```python
from build123d import *

# Parameters (mm, degrees)
EXTRUDE1_DEPTH  = 1.5875
LPATTERN2_COUNT = 5
LPATTERN2_PITCH = 0.79375


with BuildPart() as part:
    # Sketch1 → Extrude1 (new body, symmetric)
    with BuildSketch(Plane(origin=(0, 0, 0), x_dir=(1, 0, 0), z_dir=(0, 1, 0))):
        Polygon((0, 5.040989538), (-4.365625, 2.520494769), (-4.365625, -2.520494769), (0, -5.040989538), (4.365625, -2.520494769), (4.365625, 2.520494769), align=None)
    extrude(amount=EXTRUDE1_DEPTH, both=True)

    # Sketch2 → Cut-Revolve1 (revolve, cut)
    with BuildSketch(Plane(origin=(0, 0, 0), x_dir=(0, 0, -1), z_dir=(1, 0, 0))):
        Polygon((4.365625, 1.5875), (5.040989538, 1.5875), (5.040989538, 1.272572344), align=None)
    revolve(axis=Axis((0, 1.421434714, 0), (0, -1, 0)), mode=Mode.SUBTRACT)

    # Sketch3 → Cut-Revolve3 (revolve, cut)
    with BuildSketch(Plane.XY):
        Polygon((1.65317021, 1.48828125), (1.65317021, 1.5875), (0, 1.5875), (0, 0.79375), (1.65317021, 0.79375), (2.0828, 1.041796875), (2.0828, 1.240234375), align=None)
    cut_revolve3 = revolve(axis=Axis((0, 1.642101285, 0), (0, -1, 0)), mode=Mode.SUBTRACT)

    # LPattern2: Cut-Revolve3 ×5
    with Locations(*[(0, -i * LPATTERN2_PITCH, 0) for i in range(1, LPATTERN2_COUNT)]):
        add(cut_revolve3, mode=Mode.SUBTRACT)

    # Sketch4 → Cut-Revolve4 (revolve, cut)
    with BuildSketch(Plane.XY):
        Polygon((1.867985105, 1.364257812), (1.996874042, 1.5875), (1.65317021, 1.5875), (1.65317021, 1.48828125), align=None)
    revolve(axis=Axis((0, 1.785862642, 0), (0, -1, 0)), mode=Mode.SUBTRACT)

    # Sketch12 → Revolve1 (revolve)
    with BuildSketch(Plane(origin=(0, 0, 0), x_dir=(0, 0, -1), z_dir=(1, 0, 0))):
        Polygon((2.70049032, -1.7145), (3.749364928, -1.7145), (4.7625, -1.985968724), (4.631019925, -2.476659044), (3.617884853, -2.20519032), (2.0828, -2.20519032), (2.0828, -1.5875), (2.70049032, -1.5875), align=None)
    revolve(axis=Axis((0, 1.620050577, 0), (0, -1, 0)))


solid = part.part
```
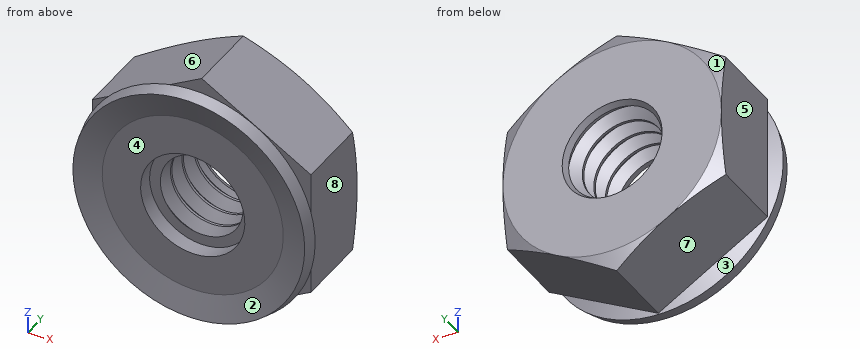
Geometry check sheet. Reference: the model listing, model coordinates, mm. Face numbers are marked on the shaded views. A direction names the side the tool comes from. Coordinates: 2 decimals unless noted, no trailing zeros. One line per item, written item: value. Start each with the question number.
(1) Depth check by flat-ended pin: pin 1 (2 mm diameter, centred on y = 0.5, z = 0, fed in from -X); pin 2 (2.5 mm diameter, centred on x = -1, z = -1.5, fed in from -Y); pin 3 (3.5 mm diameter, centred on x = 0, z = 0, fed in from -Y). Enter the tip coordinate at first touch or a pass-through.
(2) Release check for a two-part mould opening along X. For the marked faces 1, 2, 3 and 4 record: released by +X, released by -X, zero draft, split by the parting line, or undercut.
(3) Tool access check on the marked faces 5, 6, 7 and 8. Record the directions out of +Z, -Z, +X, -X, +Y, -Y that give a thin tool (end or side, any length) a straight path to the whole face; none if there is none.
(4) Scan lines: line 1 along X through (y, z) = (0.35, -2.5); line 2 along Z through (x, y) = (1.25, -0.25); line 3 along X through (y, z) = (-0.75, 0). Record each from-to range of solid material in increasing order. Write a range as [from, to].
Filled sheet:
1. pin 1: x = -4.37
1. pin 2: y = -2.21
1. pin 3: y = -1.59
2. face 1: released by -X
2. face 2: undercut
2. face 3: split by the parting line
2. face 4: undercut
3. face 5: +Z, -Z, -X, +Y
3. face 6: +Z, -X, +Y
3. face 7: -Z, -X, +Y
3. face 8: +Z, -Z, +X, +Y
4. line 1: [-4.37, 4.37]
4. line 2: [-4.32, -1.45], [1.45, 4.32]
4. line 3: [-4.37, -1.73], [1.73, 4.37]
